Job drawing, mm, ordinate dimensions from the low corner. One solid piece. A direction names the side the tool comes from. Round coordinates to 2 decimals unless told otherwise and drop trailing zeros. Write each loop counter-clockwise with the first axis right and the second up, starting at its lowest first coordinate (ties: lowest second). Pieces come first, ordered by that corner, then holes. Notation, with made-up numbers: M 58,7 L 109,7 A11 cw 109,27 Z; hole C 24.25,-20 d2. An arc over 180 degrees is marked long. Answer as a JSON object with one key per item and string values. Group by question number.
1. Which spindle directions (+Z, -Z, +X, -X, +Y, -Y) get a long thin tool onto all of the face, cutting with end or side? Do the marked faces 3 and 4. Say none if no direction does.
2. Band-saw the part on D-D, the plane x = 4.75. Write the cut outline in (y, z) (1 decimal), plus the area to 3 significant figures.
3. Two-plate mould, pull along Y, no slides. Class the marked faces 1 and 2: +Y half, -Y half, draft (parallel to the pull), parting line (faces both ways), or undercut.
4. Band-saw the part on A-A, the plane z = 60. Write the cut outline in (x, y).
5. Drill centre lines: line 1 (Z direction, x = 15.75, y = 45.5) (1 decimal); line 2 (Z direction, x = 12.5, y = 49.5) (1 decimal); line 3 (Y direction, x = 15.5, z = 68) (1 decimal). Where is each one in solid material? Low to high. Write a range as from..to.
6. Band-saw the part on C-C, the plane y = 60. Write the cut outline in (x, z).
7. Drop flat-ended pins along their axis: pin 1 (3.5 mm diameter, centred on x = 9.63, y = 59.96, fed in from +Z); pin 2 (5 mm diameter, centred on x = 9.63, y = 59.96, fed in from -Z); pin 3 (10 mm diameter, centred on x = 13, y = 78, fed in from +Z) (1 decimal); pin 4 (8 mm diameter, centred on y = 75.5, z = 67.5, fed in from -X). Give the stop position or say it passes through.
8. Band-saw the part on B-B, the plane x = 15.75. Write the cut outline in (y, z) (1 decimal), plus the area to 3 significant figures.
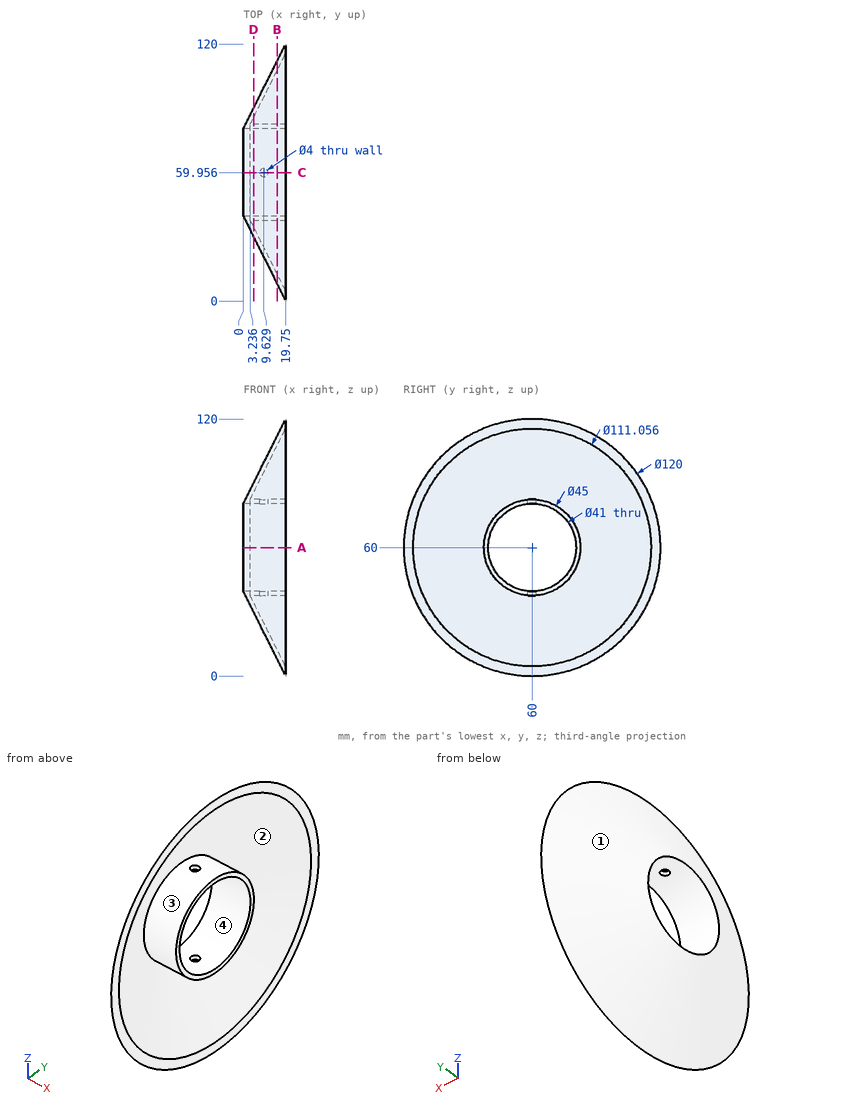
Worked answers:
{
 "1": {"face 3": "+X", "face 4": "+X, -X"},
 "2": {"outline": "C 60,60 d60; C 60,60 d45; hole C 60,60 d51.1; hole C 60,60 d41", "area": "1,050 mm^2"},
 "3": {"face 1": "parting line", "face 2": "undercut"},
 "4": {"outline": "M 0,39.5 L 19.75,0 L 19.75,4.47 L 3.24,37.5 L 19.75,37.5 L 19.75,39.5 Z; M 0,80.5 L 19.75,80.5 L 19.75,82.5 L 3.24,82.5 L 19.75,115.53 L 19.75,120 Z"},
 "5": {"line 1": "z = 10.1..14.7, 42.8..45.5, 74.5..77.2, 105.3..109.9", "line 2": "z = 15.7..20.3, 40.1..42.4, 77.6..79.9, 99.7..104.3", "line 3": "y = 9.1..13.7, 39..41.1, 78.9..81, 106.3..110.9"},
 "6": {"outline": "M 0,39.5 L 19.75,0 L 19.75,4.47 L 3.24,37.5 L 7.63,37.5 L 7.63,39.5 Z; M 0,80.5 L 7.63,80.5 L 7.63,82.5 L 3.24,82.5 L 19.75,115.53 L 19.75,120 Z; M 11.63,37.5 L 19.75,37.5 L 19.75,39.5 L 11.63,39.5 Z; M 11.63,80.5 L 19.75,80.5 L 19.75,82.5 L 11.63,82.5 Z"},
 "7": {"pin 1": "stops at z = 103.26", "pin 2": "stops at z = 15.24", "pin 3": "stops at z = 113.7", "pin 4": "stops at x = 0"},
 "8": {"outline": "C 60,60 d104; C 60,60 d45; hole C 60,60 d95.1; hole C 60,60 d41", "area": "1,670 mm^2"}
}
